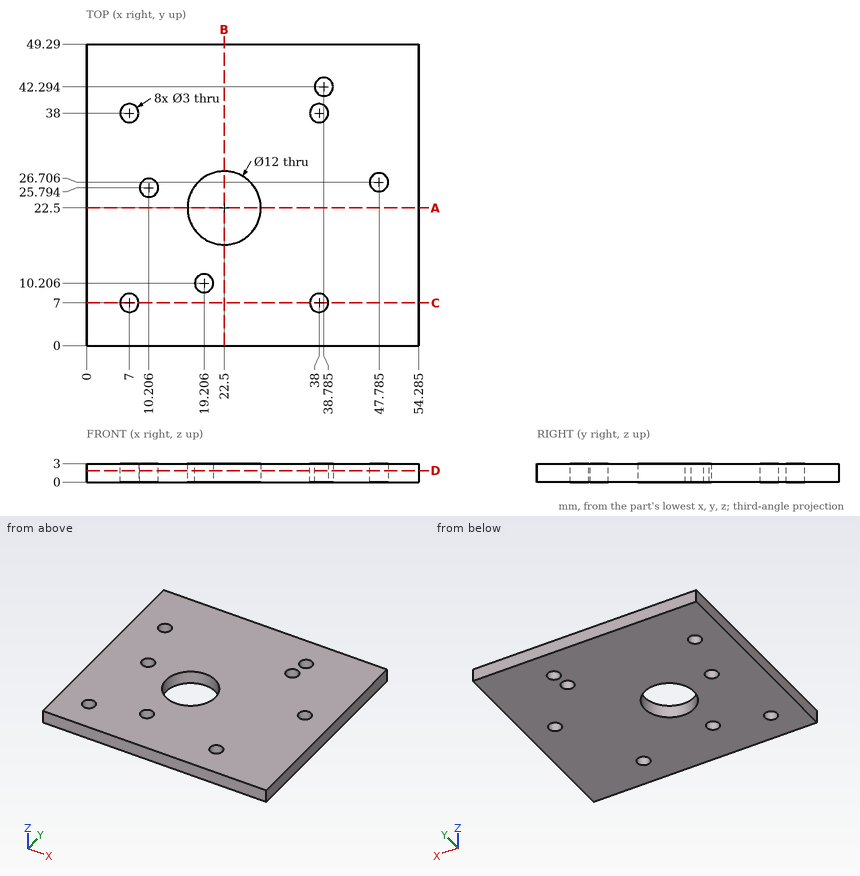
The drawing under review shows one solid part. Ordinate dimensions are in mm from its lowest x, y, z. Give positions to 0.01 mm unless a question says otherwise; leave off trailing zeros. Order: outer loops, then holes, each group sorted by start corner. A loop starts at its lowest first (then second) coordinate and runs counter-clockwise, first axis right, second up. Notation, with made-up numbers: (51, 40.25) -> (84, 40.25) arc R23 ccw to (84, 58.25) -> close; hole circle Ø2 at (16, 68). An arc over 180 degrees is marked (long way). Write item = value, one per line.
1) To check wall thickness, follow L1, parallel to Y at x = 7, z = 2.1; L2, parallel to X at y = 6, z = 2.7 (1 decimal); L3, parallel to Y at x = 22.5, z = 1.7. State the ranges of each line that lie inside material, in increasing order. Write a range as from..to.
Findings:
L1 = 0..5.5, 8.5..36.5, 39.5..49.29
L2 = 0..5.9, 8.1..36.9, 39.1..54.3
L3 = 0..16.5, 28.5..49.29
2) We need section C-C, the plane y = 7. Give the boundary of the cut face in (x, z) (1 decimal), and give its area (3 significant figures).
Findings:
outline = (0, 0) -> (5.5, 0) -> (5.5, 3) -> (0, 3) -> close; (8.5, 0) -> (36.5, 0) -> (36.5, 3) -> (8.5, 3) -> close; (39.5, 0) -> (54.3, 0) -> (54.3, 3) -> (39.5, 3) -> close
area = 145 mm^2
3) We need section B-B, the plane x = 22.5. Give the boundary of the cut face in (y, z).
Findings:
outline = (0, 0) -> (16.5, 0) -> (16.5, 3) -> (0, 3) -> close; (28.5, 0) -> (49.29, 0) -> (49.29, 3) -> (28.5, 3) -> close
4) We need section A-A, the plane y = 22.5. Give the boundary of the cut face in (x, z) (1 decimal), and give its area (3 significant figures).
Findings:
outline = (0, 0) -> (16.5, 0) -> (16.5, 3) -> (0, 3) -> close; (28.5, 0) -> (54.3, 0) -> (54.3, 3) -> (28.5, 3) -> close
area = 127 mm^2
5) Insertion check: pin 1 (1 mm diameter, centred on x = 7, y = 8.5, fed in from -Z). The pin has a flat end and moves straight along its axis. Give the tip position at first contact, or say it passes through.
Findings:
pin_1 = 0
6) We need section D-D, the plane z = 1.85. Count the separate pieces of the cut face and the enclosed holes in it, and give its area (3 significant figures).
Findings:
separate_pieces = 1
enclosed_holes = 9
area = 2,510 mm^2
